The model under review builds one solid part; all positions refer to its coordinate system, in mm. Round coordinates to 2 decimals unless told otherwise and drop trailing zeros. Order: outer loops, then holes, each group sorted by start corner. A loop starts at its lowest first (then second) coordinate and runs counter-clockwise, first axis right, second up.
```python
from build123d import *

# Parameters (mm, degrees)
F0_R     = 24.2146085631
F1_DEPTH = 101.6
F3_DEPTH = 25.4
F5_DEPTH = 25.4
F6_R     = 8.7323577449
F6_R_2   = 14.5344701606
F7_DEPTH = 254


with BuildPart() as f1:
    # F0 (on Front) → F1 (new body)
    with BuildSketch(Plane.XZ):
        Circle(F0_R)
    extrude(amount=F1_DEPTH)

    # F2 (on face) → F3 (join)
    with BuildSketch(Plane.XZ.offset(101.6)):
        with BuildLine():
            Line((-24.2146085631, 69.3517327309), (-24.2146085631, 0))
            ThreePointArc((-24.2146085631, 0), (0, 24.2146085631), (24.2146085631, 0))
            Line((24.2146085631, 0), (24.2146085631, 69.3517327309))
            ThreePointArc((24.2146085631, 69.3517327309), (0, 93.5663412939), (-24.2146085631, 69.3517327309))
        make_face()
        with BuildLine():
            ThreePointArc((24.2146085631, 0), (0, 24.2146085631), (-24.2146085631, 0))
            ThreePointArc((-24.2146085631, 0), (0, -24.2146085631), (24.2146085631, 0))
        make_face()
    extrude(amount=F3_DEPTH)

    # F4 (on face) → F5 (join)
    with BuildSketch(Plane(origin=(0, 0, 0), x_dir=(-1, 0, 0), z_dir=(0, 1, 0))):
        with BuildLine():
            ThreePointArc((23.9994246513, 74.3728801608), (-0.1075919559, 98.4102157735), (-24.2146085631, 74.3728801608))
            Line((-24.2146085631, 74.3728801608), (23.9994246513, 74.3728801608))
        make_face()
        with BuildLine():
            Line((-24.2146085631, 74.3728801608), (-24.2146085631, 0))
            ThreePointArc((-24.2146085631, 0), (-0.0350465649, 24.2145832011), (24.2145071151, 0.0700930563))
            Line((24.2145071151, 0.0700930563), (23.9994246513, 74.3728801608))
            Line((23.9994246513, 74.3728801608), (-24.2146085631, 74.3728801608))
        make_face()
        with BuildLine():
            ThreePointArc((24.2145071151, 0.0700930563), (-0.0350465649, 24.2145832011), (-24.2146085631, 0))
            ThreePointArc((-24.2146085631, 0), (0, -24.2146085631), (24.2146085631, 0))
            ThreePointArc((24.2146085631, 0), (24.2145832011, 0.0350465649), (24.2145071151, 0.0700930563))
        make_face()
    extrude(amount=F5_DEPTH)

    # F6 (on face) → F7 (cut)
    with BuildSketch(Plane.XZ.offset(127)):
        with Locations((0, 79.1887566447)):
            Circle(F6_R)
        Circle(F6_R_2)
    extrude(amount=-F7_DEPTH, mode=Mode.SUBTRACT)


solid = f1.part
```
(1) Insertion check: pin 1 (10 mm diameter, centred on x = -5, y = -66, fed in from +Z); pin 2 (5 mm diameter, centred on x = -17.5, y = -62.5, fed in from +Z); pin 3 (4 mm diameter, centred on x = -14.5, y = -111, fed in from -Z). Each pin has a flat end and moves straight along its axis. Give the tip position at first contact, or say it passes through.
Data:
pin 1: stops at z = 24.21
pin 2: stops at z = 19.01
pin 3: stops at z = -20.74
(2) Consider section C-C (y = -97). Write out the cut boundary in (x, z), and give its area (3 significant figures).
Data:
outline: circle Ø48.43 at (0, 0); hole circle Ø29.07 at (0, 0)
area: 1,180 mm2
(3) To check wall thickness, follow probe 1 along Z at (x, y) = (0, -114); probe 2 along Z at (x, y) = (0, 18); probe 3 along Y at (x, z) = (-11, 70). State the ranges of each line that lie inside material, in increasing order.
Data:
probe 1: z = -24.21 to -14.53, 14.53 to 70.46, 87.92 to 93.57
probe 2: z = -24.21 to -14.53, 14.53 to 70.46, 87.92 to 98.41
probe 3: y = -127 to -101.6, 0 to 25.4
(4) Consider section B-B (x = 0). Write out the cut boundary in (y, z), and give its area (3 significant figures).
Data:
outline: (-127, -24.21) - (25.4, -24.21) - (25.4, -14.53) - (-127, -14.53) - close; (-127, 14.53) - (25.4, 14.53) - (25.4, 70.46) - (0, 70.46) - (0, 24.21) - (-101.6, 24.21) - (-101.6, 70.46) - (-127, 70.46) - close; (-127, 87.92) - (-101.6, 87.92) - (-101.6, 93.57) - (-127, 93.57) - close; (0, 87.92) - (25.4, 87.92) - (25.4, 98.41) - (0, 98.41) - close
area: 5,710 mm2
(5) Consider section D-D (x = 19). Write out the cut boundary in (y, z).
Data:
outline: (-127, -15.01) - (25.4, -15.01) - (25.4, 89.28) - (0, 89.28) - (0, 15.01) - (-101.6, 15.01) - (-101.6, 84.36) - (-127, 84.36) - close
(6) Consider section A-A (z = -4). Write out the cut boundary in (x, y).
Data:
outline: (-23.88, -127) - (-13.97, -127) - (-13.97, 25.4) - (-23.88, 25.4) - close; (13.97, -127) - (23.88, -127) - (23.88, 25.4) - (13.97, 25.4) - close
(7) Draft analysis for pull direction Z (two halves, no side actions). For faces 1 (the cylindrical face through (0.53, -114.12, 93.56)), 2 (the flat face through (24.215, -114, 34)), 3 (the cylindrical face through (-1.137, 12.522, 87.847)), state which applies: pulls with the +Z half, pulls with the -Z half, needs draft (parallel to the pull), parting line crosses it, or undercut.
Data:
face 1: pulls with the +Z half
face 2: needs draft
face 3: undercut
